Part model, mm, in its own coordinate system. A direction names the side the tool comes from. Coordinates: 2 decimals unless noted, no trailing zeros. Order: outer loops, then holes, each group sorted by start corner. A loop starts at its lowest first (then second) coordinate and runs counter-clockwise, first axis right, second up.
from build123d import *


with BuildPart() as part:
    # Sketch4 → Revolve3 (revolve)
    with BuildSketch(Plane.XY):
        with BuildLine():
            Line((-103.075250338, 65.451422493), (55.11646874, 65.451422493))
            ThreePointArc((55.11646874, 65.451422493), (58.517447493, 64.855322935), (61.51296186, 63.138091197))
            Line((61.51296186, 63.138091197), (106.730008788, 25.510538776))
            Line((106.730008788, 25.510538776), (195.605450204, 49.82280509))
            Line((195.605450204, 49.82280509), (196.924749662, 45))
            Line((196.924749662, 45), (108.049308246, 20.687733685))
            ThreePointArc((108.049308246, 20.687733685), (105.670550773, 20.624072904), (103.531762227, 21.667204424))
            Line((103.531762227, 21.667204424), (58.3147153, 59.294756845))
            ThreePointArc((58.3147153, 59.294756845), (56.816958116, 60.153372714), (55.11646874, 60.451422493))
            Line((55.11646874, 60.451422493), (-103.075250338, 60.451422493))
            Line((-103.075250338, 60.451422493), (-103.075250338, 65.451422493))
        make_face()
    revolve(axis=Axis((196.924749662, 0, 0), (-1, 0, 0)))


solid = part.part
Q1. Pin check, flat tips, straight feed: pin 1 Ø10 at (x, y) = (8, -15.5) entering from -Z; pin 2 Ø1 at (y, z) = (-19, -22.5) entering from -X; pin 3 Ø3 at (y, z) = (-21.5, 44.5) entering from +X; pin 4 Ø4 at (x, z) = (16, -1.5) entering from -Y. Stop position of each tip, or through.
Results list:
pin 1: stops at z = -64.6
pin 2: stops at x = 93.58
pin 3: stops at x = 196.13
pin 4: stops at y = -65.45
Q2. Cut at C-C on x = 46.5. Write the cut outline in (y, z).
Results list:
outline: circle Ø130.9 at (0, 0); hole circle Ø120.9 at (0, 0)
Q3. Wall check: line 1 along Y through (x, z) = (20, 0); line 2 along Y through (x, z) = (29, 43). Give the ranges that are in metal, low to high.
Results list:
line 1: y = -65.45 to -60.45, 60.45 to 65.45
line 2: y = -49.34 to -42.49, 42.49 to 49.34
Q4. Mould opens along X. For faces 1 (the face through (-103.075, -58, 19)), 2 (the face through (141.915, 33.513, -10.554)), 3 (the face through (196.86, -9.81, 44.16)) say: pulls with the +X half, pulls with the -X half, needs draft (parallel to the pull), parting line crosses it, or undercut.
Results list:
face 1: pulls with the -X half
face 2: undercut
face 3: pulls with the +X half
Q5. Which spindle directions (+Z, -Z, +X, -X, +Y, -Y) get a long thin tool onto all of the face, cutting with end or side? Do faces 4 (the face through (104.53, 26.08, -8.21)), 5 (the face through (-25.087, -60.393, -2.658)), 6 (the face through (-22.872, -14.189, 63.895)). Say none if no direction does.
Results list:
face 4: none
face 5: -X
face 6: +X, -X
Q6. Cut at A-A on z = 0. Write the cut outline in (x, y).
Results list:
outline: (-103.08, -65.45) - (55.12, -65.45) arc R10 ccw to (61.51, -63.14) - (106.73, -25.51) - (195.61, -49.82) - (196.92, -45) - (108.05, -20.69) arc R5 ccw to (103.53, -21.67) - (58.31, -59.29) arc R5 cw to (55.12, -60.45) - (-103.08, -60.45) - close; (-103.08, 60.45) - (55.12, 60.45) arc R5 cw to (58.31, 59.29) - (103.53, 21.67) arc R5 ccw to (108.05, 20.69) - (196.92, 45) - (195.61, 49.82) - (106.73, 25.51) - (61.51, 63.14) arc R10 ccw to (55.12, 65.45) - (-103.08, 65.45) - close
